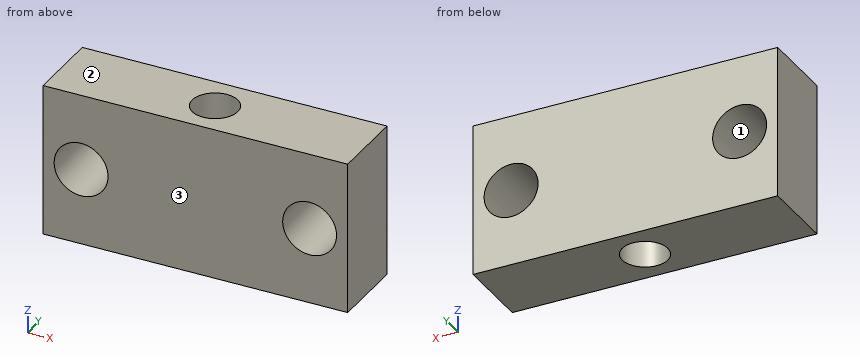
from build123d import *

# Parameters (mm, degrees)
SKETCH1_W             = 25.4
SKETCH1_H             = 12.7
BOSS_EXTRUDE1_DEPTH   = 6.35
SKETCH2_R             = 1.905
CUT_EXTRUDE1_DEPTH    = 20.05
F_8_CLEARANCE_HOLE1_D = 4.4958


with BuildPart() as part:
    # Sketch1 → Boss-Extrude1 (new body)
    with BuildSketch(Plane(origin=(0, 0, 0), x_dir=(1, 0, 0), z_dir=(0, 1, 0))):
        Rectangle(SKETCH1_W, SKETCH1_H)
    extrude(amount=BOSS_EXTRUDE1_DEPTH)

    # Sketch2 → Cut-Extrude1 (cut, through all)
    with BuildSketch(Plane(origin=(0, 0, -6.35), x_dir=(-1, 0, 0), z_dir=(0, 0, -1))):
        with Locations((0, 3.175)):
            Circle(SKETCH2_R)
    extrude(amount=-CUT_EXTRUDE1_DEPTH, mode=Mode.SUBTRACT)

    # #8 Clearance Hole1 (through all)
    with Locations(Plane(origin=(0, 6.35, 0), x_dir=(1, 0, 0), z_dir=(0, 1, 0))):
        with Locations((9.525, 0), (-9.525, 0)):
            Hole(F_8_CLEARANCE_HOLE1_D / 2)


solid = part.part
The model under review builds one solid part; all positions refer to its coordinate system, in mm. Face numbers are marked on the shaded views. Round coordinates to 2 decimals unless told otherwise and drop trailing zeros. Loops run counter-clockwise (first coordinate to the right, second up) from the corner with the lowest first, then second, coordinate; pieces in that order, holes last. Notation, with made-up numbers: (68.25, -5.5) - (113.25, -5.5) arc R21 cw to (113.25, 20.5) - close; hole circle Ø5 at (14.5, -39). An arc over 180 degrees is marked (long way). Use CSV: the item, a comma, the result in double quotes.
(1) Take a section at A-A, the plane y = 2.75. Give the boundary of the cut face in (x, z) (3 decimals).
Working result:
outline,"(-12.7, -6.35) - (-1.857, -6.35) - (-1.857, 6.35) - (-12.7, 6.35) - close; (1.857, -6.35) - (12.7, -6.35) - (12.7, 6.35) - (1.857, 6.35) - close; hole circle Ø4.496 at (-9.525, 0); hole circle Ø4.496 at (9.525, 0)"
(2) For line 1 (Y direction, x = 0, z = -2); line 2 (X direction, y = 5.5, z = 0.75); line 3 (X direction, y = 0.75, z = 2), list the stretches that pass through material, from the lowest coordinate up.
Working result:
line 1,"y = 0 to 1.27, 5.08 to 6.35"
line 2,"x = -12.7 to -11.64, -7.41 to 7.41, 11.64 to 12.7"
line 3,"x = -12.7 to -10.55, -8.5 to 8.5, 10.55 to 12.7"
(3) Take a section at B-B, the plane x = 0. Give the boundary of the cut face in (y, z), plus the area to 3 significant figures.
Working result:
outline,"(0, -6.35) - (1.27, -6.35) - (1.27, 6.35) - (0, 6.35) - close; (5.08, -6.35) - (6.35, -6.35) - (6.35, 6.35) - (5.08, 6.35) - close"
area,"32.3 mm^2"
(4) Take a section at D-D, the plane y = 6. Give the boundary of the cut face in (x, z) (3 decimals), plus the area to 3 significant figures.
Working result:
outline,"(-12.7, -6.35) - (12.7, -6.35) - (12.7, 6.35) - (-12.7, 6.35) - close; hole circle Ø4.496 at (-9.525, 0); hole circle Ø4.496 at (9.525, 0)"
area,"291 mm^2"
(5) Take a section at C-C, the plane z = 0. Give the boundary of the cut face in (x, y) (3 decimals), plus the area to 3 significant figures.
Working result:
outline,"(-12.7, 0) - (-11.773, 0) - (-11.773, 6.35) - (-12.7, 6.35) - close; (-7.277, 0) - (7.277, 0) - (7.277, 6.35) - (-7.277, 6.35) - close; (11.773, 0) - (12.7, 0) - (12.7, 6.35) - (11.773, 6.35) - close; hole circle Ø3.81 at (0, 3.175)"
area,"92.8 mm^2"
(6) The part is to be moulded in two halves that separate along Z. For the marked faces 1, 2 and 3, say which applies: pulls with the +Z half, pulls with the -Z half, needs draft (parallel to the pull), parting line crosses it, or undercut.
Working result:
face 1,"undercut"
face 2,"pulls with the +Z half"
face 3,"needs draft"
